Autodesk Inventor part; units mm, degrees
ref_plane "YZ Plane" through (0, 0, 0) normal (1, 0, 0) x (0, 1, 0)
ref_plane "XZ Plane" through (0, 0, 0) normal (0, 1, 0) x (-1, 0, 0)
ref_plane "XY Plane" through (0, 0, 0) normal (0, 0, 1) x (1, 0, 0)
sketch "Szkic1" plane through (0, 0, 0) normal (0, 1, 0) x (-1, 0, 0)
  circle A0 centre (0, 0) radius 4
  arc A1 (-2.25, -2) -> (-2.25, 2) centre (-0.75, 0) ccw
  line L0 (-2.25, 2) -> (-2.25, -2)
  dimension "d2" = 4
  dimension "d15" = 2.5
  dimension "d16" = 0.75
  dimension "d23" = 1.5
extrude "Wyciągnięcie proste1" add sketch "Szkic1" along normal blind 7
sketch "Szkic2" plane through (0, 7, 0) normal (0, 1, 0) x (1, 0, 0)
  circle A0 centre (0.75, 0) radius 6
  arc A1 (2.25, 2) -> (2.25, -2) centre (0.75, 0) ccw
  arc A2 (2.25, 2) -> (2.25, -2) centre (0.75, 0) ccw
  dimension "d32" = 6
extrude "Wyciągnięcie proste2" add sketch "Szkic2" along normal blind 1
sketch "Szkic3" plane through (0.75, 8, 0) normal (0, 1, 0) x (1, 0, 0)
  circle A0 centre (0, 0) radius 4
  circle A1 centre (0, 0) radius 6
  arc A2 (1.5, 2) -> (1.5, -2) centre (0, 0) ccw
  dimension "d33" = 4
extrude "Wyciągnięcie proste3" add sketch "Szkic3" along normal blind 3.5 contours A0
equation "\"d2\" = Lrw"
equation "\"d15\" = silnik_rw"
equation "\"d16\" = E1"
equation "\"d28\" = Lh"
equation "\"d33\" = Lrw"
equation "\"d34\" = 0.5 * Lh"
equation "\"Lrz\" = 11"
equation "\"Lrw\" = 4"
equation "\"Lh\" = 7"
equation "\"N1\" = 31"
equation "\"Rr\" = 1.5"
equation "\"R1\" = 5"
equation "\"h1\" = 2"
equation "\"h2\" = 5"
equation "\"E1\" = 0.5 * Rr"
equation "\"dwr1\" = -0.25 * Rr + 0.25 * R - 0.25 * Lrz"
equation "\"dwr2\" = 0.5 * Lrz + 0.5 * R"
equation "\"dwr\" = R"
equation "\"silnik_rw\" = 2.5"
equation "\"silnik_r_wypust\" = Lrz"
equation "\"silnik_d_srub\" = 31"
properties part number "Dysk_we"
Here's how the part is built. I have some questions about the finished solid (model axes, mm). A direction names the side the tool comes from. Round coordinates to 2 decimals unless told otherwise and drop trailing zeros. Order: outer loops, then holes, each group sorted by start corner. A loop starts at its lowest first (then second) coordinate and runs counter-clockwise, first axis right, second up. Notation, with made-up numbers: M -30,8 L 22,8 A14 cw 22,24 Z; hole C -40,51.5 d6. An arc over 180 degrees is marked long. One line per question, with ' | ' between items.
1) I want a section at B-B, the plane x = 0. Write out the boundary of the cut face in (y, z).
Working result:
outline: M 0,-4 L 7,-4 L 7,-5.95 L 8,-5.95 L 8,-3.93 L 11.5,-3.93 L 11.5,3.93 L 8,3.93 L 8,5.95 L 7,5.95 L 7,4 L 0,4 L 0,2.38 L 7,2.38 L 7,-2.38 L 0,-2.38 Z
2) If we mould it in two halves opening along X, with no side actions, what happens to faces 4 (the face through (3, 7, 3)), 5 (the face through (0, 7, 0)), 6 (the face through (0.867, 3.451, 3.905))? For each: +X half, -X half, draft (parallel to the pull), parting line (faces both ways), or undercut.
Working result:
face 4: draft | face 5: undercut | face 6: parting line
3) For faces 1 (the face through (-1.75, 3.45, 0.08)), 2 (the face through (1, 11.5, 0)), 3 (the face through (2, 8, 4)), which set-ups out of +Z, -Z, +X, -X, +Y, -Y let a thin tool reach every point of the face, with its end or its side?
Working result:
face 1: -Y | face 2: +Z, -Z, +X, -X, +Y | face 3: +Y
4) I want a section at D-D, the plane y = 1.5. Write out the boundary of the cut face in (x, z).
Working result:
outline: C 0,0 d8; hole M 2.25,-2 L 2.25,2 A2.5 ccw long Z
5) For pin 1 Ø1 at (x, y) = (-3.5, 7) entering from -Z; pin 2 Ø3 at (x, y) = (3.5, 9) entering from -Z; pin 3 Ø2 at (x, z) = (0.5, -0.5) entering from -Y, each with a flat end and sliding along its axis, tell me the tip position at first contact or that it passes through.
Working result:
pin 1: z = -4.68 | pin 2: z = -5.77 | pin 3: y = 7
6) I want a section at A-A, the plane z = 0. Write out the boundary of the cut face in (x, y).
Working result:
outline: M -5.25,7 L -4,7 L -4,0 L -1.75,0 L -1.75,7 L 2.25,7 L 2.25,0 L 4,0 L 4,7 L 6.75,7 L 6.75,8 L 4.75,8 L 4.75,11.5 L -3.25,11.5 L -3.25,8 L -5.25,8 Z
7) I need wall thicknesses on line 1 along Y through (x, z) = (0, 1); line 2 along Y through (x, z) = (-2.25, 3.25); line 3 along Z through (x, y) = (0.75, 4.75). Which ranges of each line are inside material? Lowest first, please.
Working result:
line 1: 7 to 11.5 | line 2: 0 to 8 | line 3: -3.93 to -2.5, 2.5 to 3.93
8) I want a section at C-C, the plane y = 10.25. Write out the boundary of the cut face in (x, z).
Working result:
outline: C 0.75,0 d8
